Job drawing, mm, ordinate dimensions from the low corner. One solid piece. Coordinates: 2 decimals unless noted, no trailing zeros. Write each loop counter-clockwise with the first axis right and the second up, starting at its lowest first coordinate (ties: lowest second). Pieces come first, ordered by that corner, then holes. Notation, with made-up numbers: (-12, 47.5) - (46, 47.5) arc R25 cw to (46, 80.5) - close; hole circle Ø9 at (11.25, -5.5). An arc over 180 degrees is marked (long way). Put each result on its own line as item: value. Start each with the question number.
1. Drop flat-ended pins along their axis: P1, Ø6, axis at y = 10.5, z = 5, coming from the +X side; P2, Ø2, axis at y = 10, z = 6.5, coming from the +X side. Give the stop position or say it passes through.
2. Saw through at A-A, the plane z = 6.5. Give the number of separate pieces and of enclosed holes in the cut face, plus the area to 3 significant figures.
3. Drill centre lines: L1, parallel to Y at x = 76.55, z = 8.75; L2, parallel to Y at x = 60, z = 7.5; L3, parallel to X at y = 2.75, z = 5.25. Where is each one in solid material? Low to high. Write a range as from..to.
4. Saw through at D-D, the plane y = 10.75. Write the cut outline in (x, z), plus the area to 3 significant figures.
5. Saw through at B-B, the plane x = 59.35. Write the cut outline in (y, z).
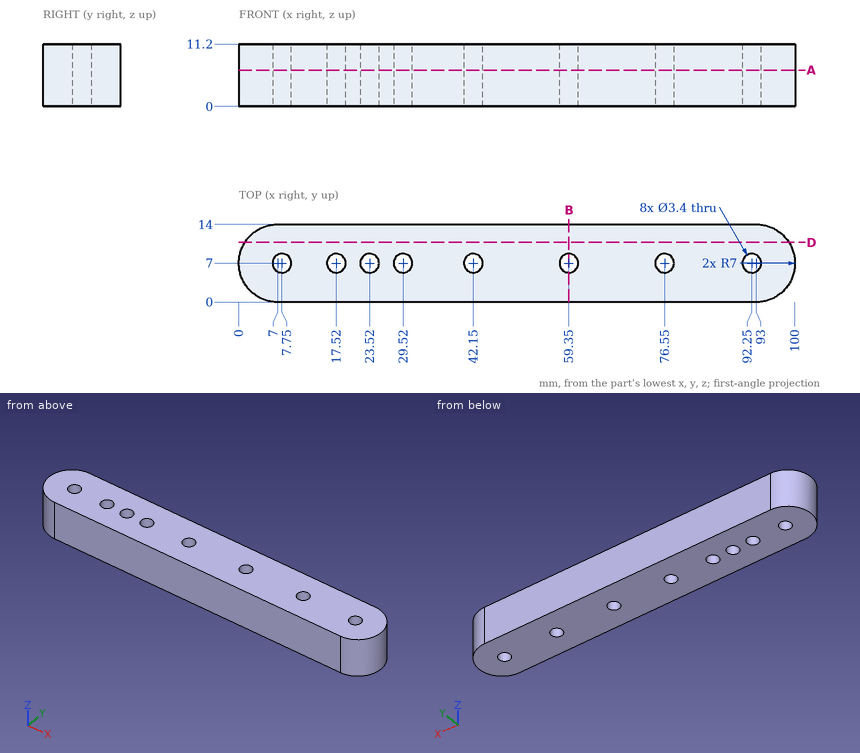
Final values:
1. P1: stops at x = 99.98
1. P2: stops at x = 99.71
2. separate pieces: 1
2. enclosed holes: 8
2. area: 1,290 mm²
3. L1: y = 0..5.3, 8.7..14
3. L2: y = 0..5.43, 8.57..14
3. L3: x = 1.44..98.56
4. outline: (1.09, 0) - (98.91, 0) - (98.91, 11.2) - (1.09, 11.2) - close
4. area: 1,100 mm²
5. outline: (0, 0) - (5.3, 0) - (5.3, 11.2) - (0, 11.2) - close; (8.7, 0) - (14, 0) - (14, 11.2) - (8.7, 11.2) - close
